Check sheet for the modelled part. Datum: model origin and axes. Units: mm. Face numbers are marked on the shaded views. Give positions to 0.01 mm unless a question says otherwise; leave off trailing zeros. Order: outer loops, then holes, each group sorted by start corner. A loop starts at its lowest first (then second) coordinate and runs counter-clockwise, first axis right, second up. Notation, with made-up numbers: (43.5, 67.25) - (62.5, 67.25) arc R8 cw to (62.5, 71.25) - close; hole circle Ø6 at (-0.75, 24). An arc over 180 degrees is marked (long way). Answer in a Markdown table with one row per item.
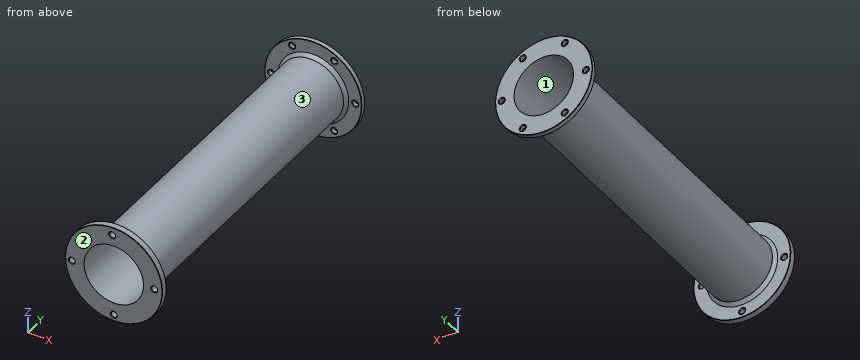
from build123d import *

# Parameters (mm, degrees)
SKIZZE1_R                       = 150
SKIZZE1_R_2                     = 92
SKIZZE1_R_3                     = 9
AUFSATZ_LINEAR_AUSTRAGEN1_DEPTH = 20
SKIZZE2_R                       = 100
SKIZZE2_R_2                     = 92
AUFSATZ_LINEAR_AUSTRAGEN2_DEPTH = 965
SKIZZE3_R                       = 150
SKIZZE3_R_2                     = 92
SKIZZE3_R_3                     = 9
AUFSATZ_LINEAR_AUSTRAGEN3_DEPTH = 15
FASE1_SIZE                      = 10
FASE2_SIZE                      = 1
FASE3_SIZE                      = 2


with BuildPart() as part:
    # Skizze1 → Aufsatz-Linear austragen1 (new body)
    with BuildSketch(Plane(origin=(0, 0, 0), x_dir=(1, 0, 0), z_dir=(0, 1, 0))):
        with Locations(Location((0, 0, 0), (0, 0, 270))):
            Circle(SKIZZE1_R)
        with Locations(Location((0, 0, 0), (0, 0, 270))):
            Circle(SKIZZE1_R_2, mode=Mode.SUBTRACT)
        with Locations(Location((0, 130, 0), (0, 0, 270))):
            Circle(SKIZZE1_R_3, mode=Mode.SUBTRACT)
        with Locations(Location((125, 0, 0), (0, 0, 270))):
            Circle(SKIZZE1_R_3, mode=Mode.SUBTRACT)
        with Locations(Location((-5, -125, 0), (0, 0, 270))):
            Circle(SKIZZE1_R_3, mode=Mode.SUBTRACT)
        with Locations(Location((-130, 5, 0), (0, 0, 270))):
            Circle(SKIZZE1_R_3, mode=Mode.SUBTRACT)
    extrude(amount=AUFSATZ_LINEAR_AUSTRAGEN1_DEPTH)

    # Skizze2 → Aufsatz-Linear austragen2 (add)
    with BuildSketch(Plane(origin=(0, 20, 0), x_dir=(1, 0, 0), z_dir=(0, 1, 0))):
        with Locations(Location((0, 0, 0), (0, 0, 270))):
            Circle(SKIZZE2_R)
        with Locations(Location((0, 0, 0), (0, 0, 270))):
            Circle(SKIZZE2_R_2, mode=Mode.SUBTRACT)
    extrude(amount=AUFSATZ_LINEAR_AUSTRAGEN2_DEPTH)

    # Skizze3 → Aufsatz-Linear austragen3 (add)
    with BuildSketch(Plane(origin=(0, 985, 0), x_dir=(1, 0, 0), z_dir=(0, 1, 0))):
        with Locations(Location((0, 0, 0), (0, 0, 270))):
            Circle(SKIZZE3_R)
        with Locations(Location((0, 0, 0), (0, 0, 270))):
            Circle(SKIZZE3_R_2, mode=Mode.SUBTRACT)
        with Locations(Location((130, 0, 0), (0, 0, 270))):
            Circle(SKIZZE3_R_3, mode=Mode.SUBTRACT)
        with Locations(Location((65, -112.583302492, 0), (0, 0, 270))):
            Circle(SKIZZE3_R_3, mode=Mode.SUBTRACT)
        with Locations(Location((-65, -112.583302492, 0), (0, 0, 270))):
            Circle(SKIZZE3_R_3, mode=Mode.SUBTRACT)
        with Locations(Location((-130, 0, 0), (0, 0, 270))):
            Circle(SKIZZE3_R_3, mode=Mode.SUBTRACT)
        with Locations(Location((-65, 112.583302492, 0), (0, 0, 270))):
            Circle(SKIZZE3_R_3, mode=Mode.SUBTRACT)
        with Locations(Location((65, 112.583302492, 0), (0, 0, 270))):
            Circle(SKIZZE3_R_3, mode=Mode.SUBTRACT)
    extrude(amount=AUFSATZ_LINEAR_AUSTRAGEN3_DEPTH)

    # Fase1
    fase1_edges = [part.edges().sort_by_distance(p)[0] for p in [
        (0, 985, -100),
        (0, 20, -100),
    ]]
    chamfer(fase1_edges, length=FASE1_SIZE)

    # Fase2
    fase2_edges = [part.edges().sort_by_distance(p)[0] for p in [
        (0, 0, -150),
        (0, 1000, -150),
        (0, 985, -150),
        (0, 20, -150),
    ]]
    chamfer(fase2_edges, length=FASE2_SIZE)

    # Fase3
    fase3_edges = [part.edges().sort_by_distance(p)[0] for p in [
        (125, 0, -9),
        (125, 20, -9),
        (-5, 0, 116),
        (-5, 20, 116),
        (-130, 0, -14),
        (-130, 20, -14),
        (130, 985, -9),
        (65, 985, 103.583302492),
        (-65, 985, 103.583302492),
        (-130, 985, -9),
        (-65, 985, -121.583302492),
        (65, 985, -121.583302492),
        (130, 1000, -9),
        (65, 1000, 103.583302492),
        (-65, 1000, 103.583302492),
        (-130, 1000, -9),
        (-65, 1000, -121.583302492),
        (65, 1000, -121.583302492),
        (0, 0, -139),
        (0, 20, -139),
    ]]
    chamfer(fase3_edges, length=FASE3_SIZE)


solid = part.part
(1) Mould release check, pull along X, two halves, no side actions. Record for the marked faces 1, 2 and 3: pulls with the +X half, pulls with the -X half, needs draft (parallel to the pull), parting line crosses it, or undercut.
Geometry says:
| item | result |
|---|---|
| face 1 | undercut |
| face 2 | needs draft |
| face 3 | parting line crosses it |
(2) Gauge pin test, flat ends, axial feed: P1, Ø4, axis at y = 299.5, z = 76, coming from the +X side; P2, Ø1, axis at y = 713.5, z = 8, coming from the -X side; P3, Ø1.5, axis at y = 490.5, z = 22.5, coming from the -X side. Record the tip position at first contact, or that the pin passes through.
Geometry says:
| item | result |
|---|---|
| P1 | x = 67.26 |
| P2 | x = -99.72 |
| P3 | x = -97.61 |
(3) Cross-section at A-A, the plane y = 152. Record the cut outline in (x, z), then the cut area to 3 significant figures.
Geometry says:
| item | result |
|---|---|
| outline | circle Ø200 at (0, 0); hole circle Ø184 at (0, 0) |
| area | 4,830 mm² |
(4) Cross-section at B-B, the plane x = -130. Give the number of separate pieces and of enclosed holes in the cut face, then the cut area to 3 significant figures.
Geometry says:
| item | result |
|---|---|
| separate pieces | 4 |
| enclosed holes | 0 |
| area | 4,580 mm² |
(5) Thickness scan on L1, parallel to X at y = 991, z = 0; L2, parallel to Y at x = 122, z = -47.5; L3, parallel to Y at x = 57, z = 106. Record the ranges inside material, lowest first.
Geometry says:
| item | result |
|---|---|
| L1 | -150 to -139, -121 to -92, 92 to 121, 139 to 150 |
| L2 | 0 to 20, 985 to 1000 |
| L3 | 0 to 20, 985.64 to 999.36 |
